Could you check a few things on this model? Use its own coordinates, in mm. A direction names the side the tool comes from. Coordinates: 2 decimals unless noted, no trailing zeros. Order: outer loops, then holes, each group sorted by start corner. A loop starts at its lowest first (then second) coordinate and runs counter-clockwise, first axis right, second up. Notation, with made-up numbers: (-0.75, -27) -> (19.25, -27) arc R24 ccw to (19.25, -3) -> close; hole circle Ø1 at (4, 69). An arc over 180 degrees is marked (long way). Return JSON: item names as keys, results as strings. Group by question number.
from build123d import *

# Parameters (mm, degrees)
F0_W     = 177.8
F0_H     = 114.3
F1_DEPTH = 57.15
F2_T     = -2.54
F4_DEPTH = 38.1


with BuildPart() as f1:
    # F0 (on Top) → F1 (new body)
    with BuildSketch(Plane.XY):
        with Locations((20.6855162978, 20.978878082)):
            Rectangle(F0_W, F0_H)
    extrude(amount=F1_DEPTH)

    # F2
    f2_openings = [f1.faces().sort_by_distance(p)[0] for p in [
        (20.685516, 20.978878, 57.15),
    ]]
    offset(amount=F2_T, openings=f2_openings)

    # F3 (on face) → F4 (join)
    with BuildSketch(Plane.XY.offset(57.15)):
        Polygon((-68.2144837022, 75.588878082), (-65.6744837022, 75.588878082), (107.0455162978, 75.588878082), (109.5855162978, 75.588878082), (109.5855162978, 78.128878082), (-68.2144837022, 78.128878082), align=None)
    extrude(amount=F4_DEPTH)


solid = f1.part
Q1. I'm going to push flat-ended pins straight in: pin 1 Ø2 at (x, y) = (58.5, 45.5) entering from +Z; pin 2 Ø12 at (x, z) = (17.5, 77.5) entering from -Y. Where does each tip first touch, or does it pass through?
Q2. On a 3-axis mill with a long thin cutter (end or side, diameter ignored), from which of +Z, -Z, +X, -X, +Y, -Y can I reach the whole of each face in a straight line? I mean faces 1 (the flat face through (20, -34, 57.15)), 2 (the flat face through (-68.214, 22, 26)), 3 (the flat face through (107.046, 20, 29)). Say none if no direction works.
Q3. I want a section at D-D on z = 73. Please give me the cut outline in (x, y), and give its area (3 significant figures).
Q4. I want a section at C-C on y = 44.5. Please give me the cut outline in (x, z).
Q5. I need wall thicknesses on line 1 along X through (y, z) = (-31, 49); line 2 along Y through (x, z) = (-59, 31.5); line 3 along Y through (x, z) = (-13, 86). Which ranges of each line are inside material? Lowest first, please. Write a range as from..to.
Q6. I want a section at B-B on x = -27.5. Please give me the cut outline in (y, z).
Q7. We'd pull the mould along Y, two halves only. Please class faces 4 (the flat face through (19, -36.171, 28)), 5 (the flat face through (109.586, 20, 26)), 6 (the flat face through (22, 78.129, 47)), 7 (the flat face through (-65.674, 20, 29)): pulls with the +Y half, pulls with the -Y half, needs draft (parallel to the pull), parting line crosses it, or undercut.
Q8. I want a section at A-A on z = 44.5. Please give me the cut outline in (x, y).
Response values:
{
 "1": {"pin 1": "stops at z = 2.54", "pin 2": "stops at y = 75.59"},
 "2": {"face 1": "+Z, +X, -X, -Y", "face 2": "+Z, -Z, -X, +Y, -Y", "face 3": "+Z"},
 "3": {"outline": "(-68.21, 75.59) -> (109.59, 75.59) -> (109.59, 78.13) -> (-68.21, 78.13) -> close", "area": "452 mm²"},
 "4": {"outline": "(-68.21, 0) -> (109.59, 0) -> (109.59, 57.15) -> (107.05, 57.15) -> (107.05, 2.54) -> (-65.67, 2.54) -> (-65.67, 57.15) -> (-68.21, 57.15) -> close"},
 "5": {"line 1": "x = -68.21..-65.67, 107.05..109.59", "line 2": "y = -36.17..-33.63, 75.59..78.13", "line 3": "y = 75.59..78.13"},
 "6": {"outline": "(-36.17, 0) -> (78.13, 0) -> (78.13, 95.25) -> (75.59, 95.25) -> (75.59, 2.54) -> (-33.63, 2.54) -> (-33.63, 57.15) -> (-36.17, 57.15) -> close"},
 "7": {"face 4": "pulls with the -Y half", "face 5": "needs draft", "face 6": "pulls with the +Y half", "face 7": "undercut"},
 "8": {"outline": "(-68.21, -36.17) -> (109.59, -36.17) -> (109.59, 78.13) -> (-68.21, 78.13) -> close; hole (-65.67, -33.63) -> (107.05, -33.63) -> (107.05, 75.59) -> (-65.67, 75.59) -> close"}
}
